The figure shows three views and two pictorial views of one solid part (mm, origin at its lowest corner). Answer the questions. A direction names the side the tool comes from. Round coordinates to 2 decimals unless told otherwise and drop trailing zeros. Order: outer loops, then holes, each group sorted by start corner. A loop starts at its lowest first (then second) coordinate and runs counter-clockwise, first axis right, second up. Notation, with made-up numbers: (-18, 65) -> (27, 65) arc R17 cw to (27, 80) -> close; hole circle Ø8 at (-20, -36). An arc over 180 degrees is marked (long way). Answer as a JSON object with one key per item and string values. Group by question number.
Item 1: Section A-A, the plane z = 25.4 is taken. Count the separate pieces of the cut face and the enclosed holes in it, plus the area to 3 significant figures.
Item 2: Section B-B, the plane z = 19 is taken. Write down the section's boundary in (x, y) (1 decimal).
Item 3: Section D-D, the plane x = 33.5 is taken. Write down the section's boundary in (y, z) (1 decimal), plus the area to 3 significant figures.
Item 4: Given P1, Ø1.2, axis at y = 6, z = 18.5, coming from the +X side; P2, Ø8, axis at x = 89, z = 14.5, coming from the +Y side (1 decimal), each flat-ended and moving along its own axis, determine where each tip first touches the part or whether it passes through.
Item 5: For the marked faces 1 and 2, determine the directions among +Z, -Z, +X, -X, +Y, -Y from which every point of the face is accessible in a straight line to the end or side of a thin tool.
Item 6: Consider probe 1 along Y at (x, z) = (83.5, 46) (1 decimal); probe 2 along X at (y, z) = (10, 20) (1 decimal); probe 3 along X at (y, z) = (2, 12.5). Determine where each line is inside the solid, lowest interval first. Write a range as from..to.
Item 7: Section C-C, the plane y = 4.25 is taken. Write down the section's boundary in (x, z).
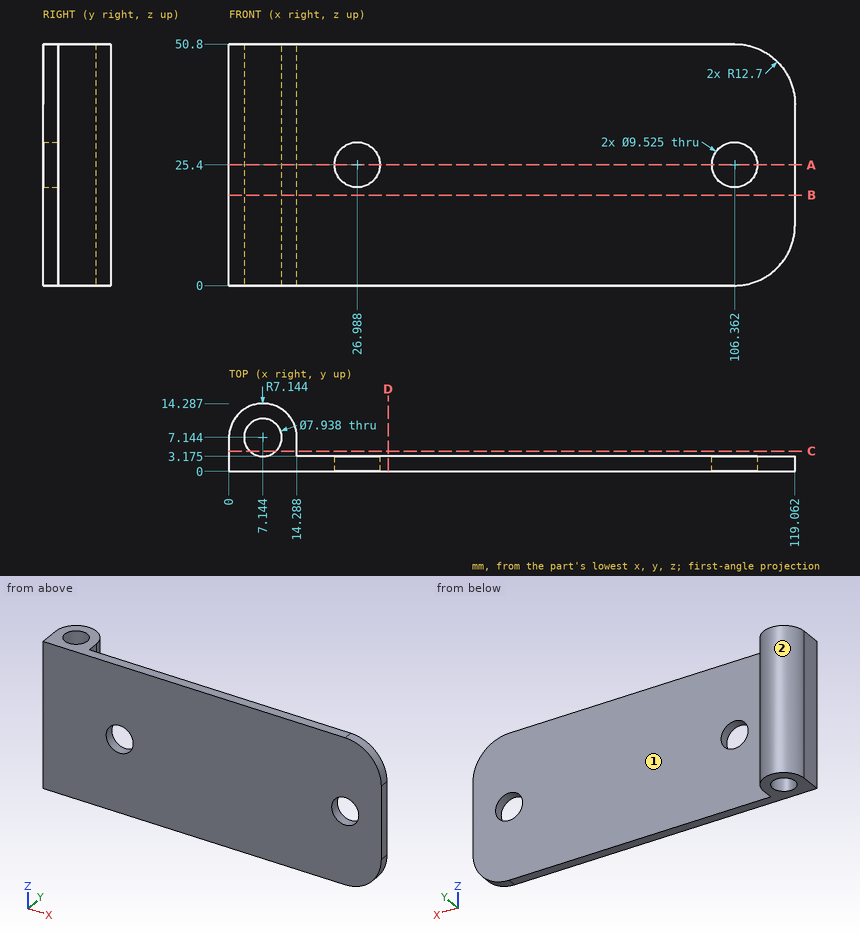
Values found:
{
 "1": {"separate pieces": "3", "enclosed holes": "1", "area": "405 mm2"},
 "2": {"outline": "(0, 0) -> (119.1, 0) -> (119.1, 3.2) -> (14.3, 3.2) -> (14.3, 7.1) arc R7.1 ccw to (0, 7.1) -> close; hole circle Ø7.9 at (7.1, 7.1)"},
 "3": {"outline": "(0, 0) -> (3.2, 0) -> (3.2, 50.8) -> (0, 50.8) -> close", "area": "161 mm2"},
 "4": {"P1": "x = 14.29", "P2": "y = 3.2"},
 "5": {"face 1": "+Z, -Z, +X, +Y", "face 2": "+Z, -Z, +Y"},
 "6": {"probe 1": "0..3.2", "probe 2": "0.6..4.4, 9.9..13.7", "probe 3": "0..119.06"},
 "7": {"outline": "(0, 0) -> (4.43, 0) -> (4.43, 50.8) -> (0, 50.8) -> close; (9.86, 0) -> (14.29, 0) -> (14.29, 50.8) -> (9.86, 50.8) -> close"}
}
